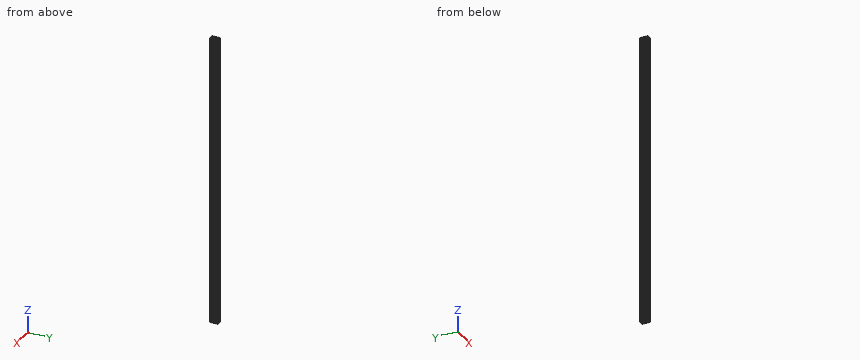
Autodesk Inventor part; units mm, degrees
ref_plane "YZ Plane" through (0, 0, 0) normal (1, 0, 0) x (0, 1, 0)
ref_plane "XZ Plane" through (0, 0, 0) normal (0, 1, 0) x (-1, 0, 0)
ref_plane "XY Plane" through (0, 0, 0) normal (0, 0, 1) x (1, 0, 0)
sketch "Sketch1" plane through (0, 0, 0) normal (0, 0, 1) x (1, 0, 0)
  line L0 (-3.9007, 3.9007) -> (3.9007, 3.9007)
  line L1 (3.9007, 3.9007) -> (3.9007, -3.9007)
  line L2 (3.9007, -3.9007) -> (-3.9007, -3.9007)
  line L3 (-3.9007, -3.9007) -> (-3.9007, 3.9007)
  line L4 (0, 3.9007) -> (0, -3.9007) construction
  line L5 (-3.9007, 0) -> (3.9007, 0) construction
  circle A0 centre (0, 0) radius 2.1
  line L6 (0, 0) -> (-16.1173, 16.1173) construction
  line L7 (0, 0) -> (22.7933, 0) construction
  line L8 (-2.84, 3.9007) -> (-5.4993, 6.56)
  line L9 (-5.4993, 6.56) -> (-5.4993, 8.2)
  line L10 (-5.4993, 8.2) -> (-2.84, 8.2)
  line L11 (-2.84, 8.2) -> (-4.64, 10)
  line L12 (-4.64, 10) -> (-10, 10)
  line L13 (-10, 10) -> (-10, 4.64)
  line L14 (-10, 4.64) -> (-8.2, 2.84)
  line L15 (-8.2, 2.84) -> (-8.2, 5.4993)
  line L16 (-8.2, 5.4993) -> (-6.56, 5.4993)
  line L17 (-6.56, 5.4993) -> (-3.9007, 2.84)
  line L18 (-3.9007, 2.84) -> (-11.3102, 2.84) construction
  line L19 (-2.84, 3.9007) -> (-3.9007, 3.9007)
  line L20 (-3.9007, 2.84) -> (-3.9007, 3.9007)
  line L21 (-3.9007, -2.84) -> (-6.56, -5.4993)
  line L22 (-6.56, -5.4993) -> (-8.2, -5.4993)
  line L23 (-8.2, -5.4993) -> (-8.2, -2.84)
  line L24 (-8.2, -2.84) -> (-10, -4.64)
  line L25 (-10, -4.64) -> (-10, -10)
  line L26 (-10, -10) -> (-4.64, -10)
  line L27 (-4.64, -10) -> (-2.84, -8.2)
  line L28 (-2.84, -8.2) -> (-5.4993, -8.2)
  line L29 (-5.4993, -8.2) -> (-5.4993, -6.56)
  line L30 (-5.4993, -6.56) -> (-2.84, -3.9007)
  line L31 (-3.9007, -2.84) -> (-3.9007, -3.9007)
  line L32 (-2.84, -3.9007) -> (-3.9007, -3.9007)
  line L33 (2.84, -3.9007) -> (5.4993, -6.56)
  line L34 (5.4993, -6.56) -> (5.4993, -8.2)
  line L35 (5.4993, -8.2) -> (2.84, -8.2)
  line L36 (2.84, -8.2) -> (4.64, -10)
  line L37 (4.64, -10) -> (10, -10)
  line L38 (10, -10) -> (10, -4.64)
  line L39 (10, -4.64) -> (8.2, -2.84)
  line L40 (8.2, -2.84) -> (8.2, -5.4993)
  line L41 (8.2, -5.4993) -> (6.56, -5.4993)
  line L42 (6.56, -5.4993) -> (3.9007, -2.84)
  line L43 (2.84, -3.9007) -> (3.9007, -3.9007)
  line L44 (3.9007, -2.84) -> (3.9007, -3.9007)
  line L45 (3.9007, 2.84) -> (6.56, 5.4993)
  line L46 (6.56, 5.4993) -> (8.2, 5.4993)
  line L47 (8.2, 5.4993) -> (8.2, 2.84)
  line L48 (8.2, 2.84) -> (10, 4.64)
  line L49 (10, 4.64) -> (10, 10)
  line L50 (10, 10) -> (4.64, 10)
  line L51 (4.64, 10) -> (2.84, 8.2)
  line L52 (2.84, 8.2) -> (5.4993, 8.2)
  line L53 (5.4993, 8.2) -> (5.4993, 6.56)
  line L54 (5.4993, 6.56) -> (2.84, 3.9007)
  line L55 (3.9007, 2.84) -> (3.9007, 3.9007)
  line L56 (2.84, 3.9007) -> (3.9007, 3.9007)
  dimension "d7" = 4.2
  dimension "d8" = 135
  dimension "d9" = 1.5
  dimension "d10" = 1.64
  dimension "d11" = 1.8
  dimension "d12" = 2.84
  dimension "d13" = 10
  dimension "d16" = 360
extrude "Extrusion1" add sketch "Sketch1" along normal blind 1500
pattern_linear "Rectangular Pattern1" count 2 spacing 20 along (0, -1, 0) of "Extrusion1"
sketch "Sketch2" plane through (0, 0, 1500) normal (0, 0, 1) x (1, 0, 0)
  line L0 (8.2, -2.84) -> (8.2, -5.4993)
  line L1 (8.2, -5.4993) -> (6.56, -5.4993)
  line L2 (-6.56, -5.4993) -> (-8.2, -5.4993)
  line L3 (-8.2, -5.4993) -> (-8.2, -2.84)
  line L4 (-8.2, -14.5007) -> (-6.56, -14.5007)
  line L5 (6.56, -14.5007) -> (8.2, -14.5007)
  line L6 (5.4993, -11.8) -> (5.4993, -13.44)
  line L7 (5.4993, -13.44) -> (2.84, -16.0993)
  line L8 (-2.84, -16.0993) -> (-5.4993, -13.44)
  line L9 (-5.4993, -8.2) -> (-5.4993, -6.56)
  line L10 (-5.4993, -6.56) -> (-2.84, -3.9007)
  line L11 (2.84, -3.9007) -> (5.4993, -6.56)
  line L12 (2.84, -8.2) -> (4.64, -10)
  line L13 (-8.2, -6.9993) -> (-5.9387, -6.9993)
  line L14 (-5.9387, -6.9993) -> (-4.1231, -5.1837)
  line L15 (-4.1231, -5.1837) -> (4.1231, -5.1837)
  line L16 (4.1231, -5.1837) -> (5.9387, -6.9993)
  line L17 (5.9387, -6.9993) -> (8.2, -6.9993)
  line L18 (8.2, -6.9993) -> (8.2, -13.0007)
  line L19 (8.2, -13.0007) -> (5.9387, -13.0007)
  line L20 (5.9387, -13.0007) -> (4.2461, -14.6932)
  line L21 (4.2461, -14.6932) -> (-4.2461, -14.6932)
  line L22 (-4.2461, -14.6932) -> (-5.9387, -13.0007)
  line L23 (-5.9387, -13.0007) -> (-8.2, -13.0007)
  line L24 (-8.2, -13.0007) -> (-8.2, -6.9993)
  dimension "d23" = 1.5
  dimension "d24" = 1.5
  dimension "d25" = 1.5
  dimension "d26" = 1.5
extrude "Extrusion2" cut sketch "Sketch2" against normal up to next
equation "\"d24\" = d23"
equation "\"d25\" = d23"
equation "\"d26\" = d23"
properties part number "20x40x1500mm"
The model under review builds one solid part; all positions refer to its coordinate system, in mm. Round coordinates to 2 decimals unless told otherwise and drop trailing zeros. Use CSV: the item, a comma, the result in double quotes.
(1) Clearance check with flat-ended pins moving along their axes: P1, Ø10, axis at x = 4, y = -24, coming from the -Z side; P2, Ø3, axis at x = -1.5, z = 995, coming from the -Y side; P3, Ø3, axis at x = -1, z = 388, coming from the -Y side; P4, Ø2, axis at y = -23.5, z = 887.5, coming from the -X side. State where each tip first meets the part, or that it passes through.
Working result:
P1,"stops at z = 0"
P2,"stops at y = -28.36"
P3,"stops at y = -23.9"
P4,"stops at x = -9.86"
(2) For line 1 (Y direction, x = -1, z = 255); line 2 (Y direction, x = 0, z = 1037.5); line 3 (X direction, y = -25, z = 899), list the stretches that pass through material, from the lowest coordinate up.
Working result:
line 1,"y = -23.9 to -21.85, -18.15 to -16.1, -3.9 to -1.85, 1.85 to 3.9"
line 2,"y = -23.9 to -22.1, -17.9 to -16.1, -3.9 to -2.1, 2.1 to 3.9"
line 3,"x = -10 to -8.2, -6.06 to -3.94, 3.94 to 6.06, 8.2 to 10"
(3) Take a section at A-A, the plane z = 1068. State how many separate pieces and enclosed holes the cut face has, plus the area to 3 significant figures.
Working result:
separate pieces,"1"
enclosed holes,"3"
area,"297 mm^2"
